from build123d import *

# Parameters (mm, degrees)
F1_W     = 32
F1_H     = 21.1428571429
F2_DEPTH = 4.5714285714
F3_SIZE2 = 2.5477916399
F3_SIZE  = 7
F4_R     = 1
F5_DEPTH = 3


with BuildPart() as f2:
    # F1 (on Top) → F2 (new body)
    with BuildSketch(Plane.XY):
        with Locations((16, -10.5714285714)):
            Rectangle(F1_W, F1_H)
    extrude(amount=F2_DEPTH)

    # F3
    f3_edges = [f2.edges().sort_by_distance(p)[0] for p in [
        (0, -10.571429, 4.571429),
        (16, -21.142857, 4.571429),
        (32, -10.571429, 4.571429),
    ]]
    f3_side = f2.faces().sort_by_distance((16, -10.571429, 4.571429))[0]
    chamfer(f3_edges, length=F3_SIZE, length2=F3_SIZE2, reference=f3_side)

    # F4 (on face) → F5 (cut)
    with BuildSketch(Plane.XY.offset(4.5714285714)):
        with Locations((16, -7.0714285714)):
            Circle(F4_R)
    extrude(amount=-F5_DEPTH, mode=Mode.SUBTRACT)


solid = f2.part
Input: part model. Units: mm. Frame: model coordinates. A direction names the side the tool comes from. Give positions to 0.01 mm unless a question says otherwise; leave off trailing zeros. Write each loop counter-clockwise with the first axis right and the second up, starting at its lowest first coordinate (ties: lowest second). Pieces come first, ordered by that corner, then holes. Notation, with made-up numbers: (-1, -27) -> (53, -27) arc R30 ccw to (53, 7) -> close; hole circle Ø2 at (32.5, 19.5). An arc over 180 degrees is marked (long way). Use one line per item in the form item = value. Start each with the question number.
1) Section query C-C on z = 3.1. Return the cut outline in (x, y).
2) Set-up query: faces 1 (the cylindrical face through (16.924, -7.454, 3.092)), 2 (the flat face through (16, 0, 2)). Return all of +Z, -Z, +X, -X, +Y, -Y with unobstructed straight access to the full face (end or side cutting, diameter ignored); none if empty.
3) Section query D-D on x = 16. Return the cut outline in (y, z).
4) Section query A-A on y = -11. Return the cut outline in (x, z).
5) Section query B-B on x = 20. Return the cut outline in (y, z).
6) Draft query along X for faces 3 (the flat face through (16, -21.143, 1)), 4 (the flat face through (16, -7, 1.571)), 5 (the flat face through (0, -11, 1)). Return one class per face: pulls with the +X half, pulls with the -X half, needs draft (parallel to the pull), parting line crosses it, or undercut.
7) Pin query (flat end, axial travel): pin 1 (1.6 mm diameter, centred on x = 16, y = -7, fed in from +Z). Return the tip coordinate at first contact, or that it passes through.
8) Ray query, probe 1 along Z at (x, y) = (2.5, -6.5); probe 2 along Z at (x, y) = (30, -16.5). Return the intervals inside material, ascending. Write a range as from..to.
Outcome:
q1.outline = (2.96, -18.19) -> (29.04, -18.19) -> (29.04, 0) -> (2.96, 0) -> close; hole circle Ø2 at (16, -7.07)
q2.face_1 = +Z
q2.face_2 = +Z, -Z, +X, -X, +Y
q3.outline = (-21.14, 0) -> (0, 0) -> (0, 4.57) -> (-6.07, 4.57) -> (-6.07, 1.57) -> (-8.07, 1.57) -> (-8.07, 4.57) -> (-14.14, 4.57) -> (-21.14, 2.02) -> close
q4.outline = (0, 0) -> (32, 0) -> (32, 2.02) -> (25, 4.57) -> (7, 4.57) -> (0, 2.02) -> close
q5.outline = (-21.14, 0) -> (0, 0) -> (0, 4.57) -> (-14.14, 4.57) -> (-21.14, 2.02) -> close
q6.face_3 = needs draft
q6.face_4 = undercut
q6.face_5 = pulls with the -X half
q7.pin_1 = 1.57
q8.probe_1 = 0..2.93
q8.probe_2 = 0..2.75
